Can you work these out from the model? Positions are in its coordinate system, mm. A direction names the side the tool comes from. Round coordinates to 2 decimals unless told otherwise and drop trailing zeros. Write each loop counter-clockwise with the first axis right and the second up, starting at its lowest first coordinate (ties: lowest second). Pieces come first, ordered by that corner, then holes. Notation, with made-up numbers: (33, 35) -> (50, 35) arc R20 ccw to (50, 67) -> close; hole circle Ø10 at (40.25, 11.25). An arc over 180 degrees is marked (long way). Write item = value, one per line. Start each with the question number.
1) I'm going to push flat-ended pins straight in: pin 1 (4 mm diameter, centred on x = -2.5, y = 11, fed in from +Z); pin 2 (3 mm diameter, centred on y = 11.5, z = 0.5, fed in from -X) (3 decimals); pin 3 (2 mm diameter, centred on y = 18.5, z = 2.5, fed in from -X) (3 decimals); pin 4 (1.5 mm diameter, centred on x = 1.5, z = -2, fed in from -Y). Where does each tip first touch, or does it pass through?
2) If I drill on line 1 (Y direction, x = -0.5, z = -2.5); line 2 (Y direction, x = -2, z = 3.5); line 3 (X direction, y = 6.5, z = 0) (3 decimals), over which ranges is the centre line in solid material (lowest first)?
3) Imagine slicing it at C-C, the plane y = 15. Please give me the cut outline in (x, z) (3 decimals).
4) Imagine slicing it at B-B, the plane y = 2.75. Please give me the cut outline in (x, z), then the cut area to 3 significant figures.
5) For faces 1 (the face through (-1.873, 16.476, -0.082)), 2 (the face through (0, 27.25, 0)), which set-ups out of +Z, -Z, +X, -X, +Y, -Y let a thin tool reach every point of the face, with its end or its side?
from build123d import *

# Parameters (mm, degrees)
BOSS_EXTRUDE1_DEPTH = 6
SKETCH2_R           = 1.875
BOSS_EXTRUDE2_DEPTH = 21.25


with BuildPart() as part:
    # Sketch1 → Boss-Extrude1 (new body)
    with BuildSketch(Plane(origin=(0, 0, 0), x_dir=(1, 0, 0), z_dir=(0, 1, 0))):
        Polygon((4.618802154, 0), (2.309401077, 4), (-2.309401077, 4), (-4.618802154, 0), (-2.309401077, -4), (2.309401077, -4), align=None)
    extrude(amount=BOSS_EXTRUDE1_DEPTH)

    # Sketch2 → Boss-Extrude2 (add)
    with BuildSketch(Plane(origin=(0, 6, 0), x_dir=(1, 0, 0), z_dir=(0, 1, 0))):
        Circle(SKETCH2_R)
    extrude(amount=BOSS_EXTRUDE2_DEPTH)

    # Sketch3 → Cut-Revolve1 (revolve, cut)
    with BuildSketch(Plane.XY):
        with BuildLine():
            Line((4.618802154, 0), (3.618802154, 0))
            ThreePointArc((3.618802154, 0), (4.325908935, 0.292893219), (4.618802154, 1))
            Line((4.618802154, 1), (4.618802154, 0))
        make_face()
        with BuildLine():
            Line((4.618802154, 5), (4.618802154, 6))
            Line((4.618802154, 6), (3.618802154, 6))
            ThreePointArc((3.618802154, 6), (4.325908935, 5.707106781), (4.618802154, 5))
        make_face()
    revolve(axis=Axis((0, 0, 0), (0, -1, 0)), mode=Mode.SUBTRACT)


solid = part.part
Reported:
q1.pin_1 = 1.81
q1.pin_2 = -1.875
q1.pin_3 = -1.125
q1.pin_4 = 0
q2.line_1 = 0 to 6
q2.line_2 = 0.09 to 5.91
q2.line_3 = -1.875 to 1.875
q3.outline = circle Ø3.75 at (0, 0)
q4.outline = (-4.62, 0) -> (-2.31, -4) -> (2.31, -4) -> (4.62, 0) -> (2.31, 4) -> (-2.31, 4) -> close
q4.area = 55.4 mm²
q5.face_1 = +Y
q5.face_2 = +Z, -Z, +X, -X, +Y
